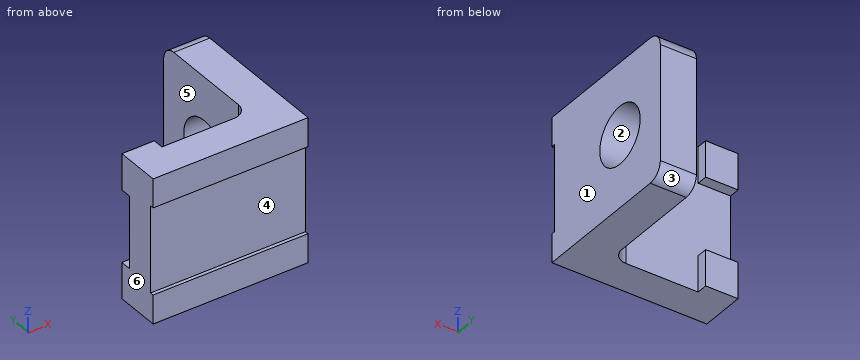
Autodesk Inventor part; units mm, degrees
ref_plane "YZ Plane" through (0, 0, 0) normal (1, 0, 0) x (0, 1, 0)
ref_plane "XZ Plane" through (0, 0, 0) normal (0, 1, 0) x (-1, 0, 0)
ref_plane "XY Plane" through (0, 0, 0) normal (0, 0, 1) x (1, 0, 0)
sketch "Sketch1" plane through (0, 0, 0) normal (0, 0, 1) x (1, 0, 0)
  line L0 (0, 0) -> (136.525, 0)
  line L1 (136.525, 0) -> (136.525, 136.525)
  line L2 (136.525, 136.525) -> (104.775, 136.525)
  line L3 (104.775, 136.525) -> (104.775, 42.545)
  line L4 (92.075, 29.845) -> (28.575, 29.845)
  line L5 (28.575, 29.845) -> (28.575, 39.37)
  line L6 (28.575, 39.37) -> (0, 39.37)
  line L7 (0, 39.37) -> (0, 0)
  arc A0 (92.075, 29.845) -> (104.775, 42.545) centre (92.075, 42.545) ccw
  point P0 (104.775, 29.845)
  dimension "d0" = 136.525
  dimension "d1" = 136.525
  dimension "d2" = 31.75
  dimension "d3" = 9.525
  dimension "d4" = 39.37
  dimension "d5" = 76.2
  dimension "d17" = 12.7
extrude "Extrusion1" add sketch "Sketch1" against normal blind 127
sketch "Sketch2" plane through (0, 39.37, 0) normal (0, 1, 0) x (1, 0, 0)
  line L0 (28.575, 0) -> (28.575, 127)
  line L1 (28.575, 95.25) -> (0, 95.25)
  line L2 (0, 95.25) -> (0, 31.75)
  line L3 (0, 0) -> (0, 127)
  line L4 (0, 31.75) -> (28.575, 31.75)
  line L5 (0, 127) -> (28.575, 127)
  dimension "d9" = 63.5
  dimension "d10" = 31.75
extrude "Extrusion2" cut sketch "Sketch2" against normal blind 9.525 contours L4 L2 L1 L0
sketch "Sketch3" plane through (0, 0, 0) normal (0, -1, 0) x (1, 0, 0)
  line L0 (0, 0) -> (0, -127)
  line L1 (0, -101.6) -> (136.525, -101.6)
  line L2 (136.525, 0) -> (136.525, -127)
  line L3 (136.525, -25.4) -> (0, -25.4)
  line L4 (0, 0) -> (136.525, 0)
  dimension "d13" = 76.2
  dimension "d14" = 25.4
extrude "Extrusion3" cut sketch "Sketch3" against normal blind 3.175 contours L3 L2 L1 L0
sketch "Sketch4" plane through (104.775, 29.845, 0) normal (-1, 0, 0) x (0, 0, 1)
  point P0 (0, -29.845)
sketch "Sketch5" plane through (104.775, 42.545, 0) normal (-1, 0, 0) x (0, 0, 1)
  circle A0 centre (-63.5, 43.18) radius 25.4
  line L0 (-127, 0) -> (-127, 93.98)
  line L1 (0, 93.98) -> (-127, 93.98)
  point P0 (0, -42.545)
  dimension "d18" = 50.8
  dimension "d19" = 63.5
  dimension "d20" = 50.8
extrude "Extrusion4" cut sketch "Sketch5" against normal through all
sketch "Sketch6" plane through (104.775, 42.545, 0) normal (-1, 0, 0) x (0, 0, 1)
  point P0 (0, -42.545)
sketch "Sketch7" plane through (104.775, 42.545, 0) normal (-1, 0, 0) x (0, 0, 1)
  point P0 (0, -42.545)
fillet "Fillet1" radius 12.7 1 edges at (120.65, 136.525, 0)
fillet "Fillet2" radius 12.7 1 edges at (120.65, 136.525, -127)
properties part number "HW 4 Part 2"
Work out the finished part from the listing and answer in its coordinate system (mm). Face numbers are marked on the shaded views. A direction names the side the tool comes from. Coordinates: 2 decimals unless noted, no trailing zeros. Loops run counter-clockwise (first coordinate to the right, second up) from the corner with the lowest first, then second, coordinate; pieces in that order, holes last. Notation, with made-up numbers: (-10.75, 36) -> (28.25, 36) arc R5 ccw to (28.25, 45) -> close; hole circle Ø11 at (28.25, -37.75). An arc over 180 degrees is marked (long way). Answer as CSV lines item,"result".
1) For the marked faces 4, 5 and 6, determine the directions among +Z, -Z, +X, -X, +Y, -Y from which every point of the face is accessible in a straight line to the end or side of a thin tool.
A:
face 4,"+X, -X, -Y"
face 5,"+Z, -Z, -X, +Y"
face 6,"+Z, -Z, -X, +Y, -Y"
2) The part is cut by section D-D (x = 86). Give the vertices of the cut face in (y, z) (3 decimals).
A:
outline,"(0, -127) -> (29.845, -127) -> (29.845, 0) -> (0, 0) -> (0, -25.4) -> (3.175, -25.4) -> (3.175, -101.6) -> (0, -101.6) -> close"
3) Flat-ended cylindrical pins translate along their axes: pin 1 (10 mm diameter, centred on x = 82.5, z = -56.5, fed in from +Y) (3 decimals); pin 2 (8.5 mm diameter, centred on x = 8, z = -114, fed in from +Y); pin 3 (1.5 mm diameter, centred on x = 107, z = -72.5, fed in from -Y) (3 decimals). Find the tip coordinate at first contact, or state that the pin passes through.
A:
pin 1,"stops at y = 29.845"
pin 2,"stops at y = 39.37"
pin 3,"stops at y = 3.175"
4) For a pull along Y with two mould halves and no side action, classify the marked faces 1, 2 and 3 as released by +Y, released by -Y, zero draft, split by the parting line, or undercut.
A:
face 1,"zero draft"
face 2,"undercut"
face 3,"released by +Y"
5) The part is cut by section A-A (z = -63.5). Give the vertices of the cut face in (x, y) (3 decimals).
A:
outline,"(0, 3.175) -> (136.525, 3.175) -> (136.525, 60.325) -> (104.775, 60.325) -> (104.775, 42.545) arc R12.7 cw to (92.075, 29.845) -> (0, 29.845) -> close; (104.775, 111.125) -> (136.525, 111.125) -> (136.525, 136.525) -> (104.775, 136.525) -> close"
6) The part is cut by section B-B (z = -20). Give the vertices of the cut face in (x, y) (3 decimals).
A:
outline,"(0, 0) -> (136.525, 0) -> (136.525, 136.525) -> (104.775, 136.525) -> (104.775, 42.545) arc R12.7 cw to (92.075, 29.845) -> (28.575, 29.845) -> (28.575, 39.37) -> (0, 39.37) -> close"
7) Straight lines are drawn through the part: probe 1 along Y at (x, z) = (111, -63.5) (3 decimals); probe 2 along Y at (x, z) = (18, -72.5) (3 decimals); probe 3 along Y at (x, z) = (57, -114) (3 decimals). For each, find the intervals that lie inside material, in ascending order.
A:
probe 1,"y = 3.175 to 60.325, 111.125 to 136.525"
probe 2,"y = 3.175 to 29.845"
probe 3,"y = 0 to 29.845"
8) The part is cut by section C-C (y = 79). Give the vertices of the cut face in (x, z) (3 decimals), and give its area (3 significant figures).
A:
outline,"(104.775, -127) -> (136.525, -127) -> (136.525, -87.994) -> (104.775, -87.994) -> close; (104.775, -39.006) -> (136.525, -39.006) -> (136.525, 0) -> (104.775, 0) -> close"
area,"2,480 mm²"
